```python
from build123d import *

# Parameters (mm, degrees)
SKETCH1_W           = 20
SKETCH1_H           = 80
BOSS_EXTRUDE1_DEPTH = 20
SKETCH2_R           = 5
CUT_EXTRUDE1_DEPTH  = 49.989794856
SKETCH5_R           = 3.175
CUT_EXTRUDE4_DEPTH  = 49.989794856
CUT_EXTRUDE3_DEPTH  = 5


with BuildPart() as part:
    # Sketch1 → Boss-Extrude1 (new body)
    with BuildSketch(Plane(origin=(0, 0, 0), x_dir=(1, 0, 0), z_dir=(0, 1, 0))):
        Rectangle(SKETCH1_W, SKETCH1_H)
    extrude(amount=BOSS_EXTRUDE1_DEPTH)

    # Sketch2 → Cut-Extrude1 (cut, through all)
    with BuildSketch(Plane(origin=(10, 0, 0), x_dir=(0, 0, -1), z_dir=(1, 0, 0))):
        with Locations((-20, 10)):
            Circle(SKETCH2_R)
        with Locations(Location((20, 10, 0), (0, 0, 180))):
            Circle(SKETCH2_R)
    extrude(amount=-CUT_EXTRUDE1_DEPTH, mode=Mode.SUBTRACT)

    # Sketch5 → Cut-Extrude4 (cut, through all)
    with BuildSketch(Plane(origin=(10, 0, 0), x_dir=(0, 0, -1), z_dir=(1, 0, 0))):
        with Locations((0, 10)):
            Circle(SKETCH5_R)
    extrude(amount=-CUT_EXTRUDE4_DEPTH, mode=Mode.SUBTRACT)

    # Sketch3 → Cut-Extrude3 (cut)
    with BuildSketch(Plane(origin=(10, 0, 0), x_dir=(0, 0, -1), z_dir=(1, 0, 0))):
        Polygon((0, 16), (-5.196152423, 13), (-5.196152423, 7), (0, 4), (5.196152423, 7), (5.196152423, 13), align=None)
    cut_extrude3 = extrude(amount=-CUT_EXTRUDE3_DEPTH, mode=Mode.SUBTRACT)

    # Mirror1: Cut-Extrude3 across plane
    add(cut_extrude3.mirror(Plane(origin=(0, 0, 0), x_dir=(0, 0, 1), z_dir=(1, 0, 0))), mode=Mode.SUBTRACT)


solid = part.part
```
The model under review builds one solid part; all positions refer to its coordinate system, in mm. A direction names the side the tool comes from. Give positions to 0.01 mm unless a question says otherwise; leave off trailing zeros. Write each loop counter-clockwise with the first axis right and the second up, starting at its lowest first coordinate (ties: lowest second). Pieces come first, ordered by that corner, then holes. Notation, with made-up numbers: (-27.5, -17.75) -> (5.5, -17.75) arc R18 ccw to (5.5, 1.25) -> close; hole circle Ø5 at (-39.75, 50.25). An arc over 180 degrees is marked (long way). Put each result on its own line as item: value.
(1) For pin 1 Ø3 at (y, z) = (9.5, -2) entering from +X; pin 2 Ø8.5 at (y, z) = (10.5, -0.5) entering from -X, all flat-tipped, find the tip position at first contact; note any pin that passes through.
Results are:
pin 1: x = 5
pin 2: x = -5
(2) Tool access review of faces 4 (the flat face through (-8, 10, -5.196)), 5 (the flat face through (-10, 3, 1)), 6 (the flat face through (7.5, 14.5, -2.6)): name each direction out of +Z, -Z, +X, -X, +Y, -Y from which nothing blocks a thin tool from reaching the whole face with its end or side.
Results are:
face 4: -X
face 5: +Z, -Z, -X, +Y, -Y
face 6: +X
(3) We need section A-A, the plane y = 10. Give the boundary of the cut face in (x, z) (3 decimals), and give its area (3 significant figures).
Results are:
outline: (-10, -40) -> (10, -40) -> (10, -25) -> (-10, -25) -> close; (-10, -15) -> (10, -15) -> (10, -5.196) -> (5, -5.196) -> (5, -3.175) -> (-5, -3.175) -> (-5, -5.196) -> (-10, -5.196) -> close; (-10, 5.196) -> (-5, 5.196) -> (-5, 3.175) -> (5, 3.175) -> (5, 5.196) -> (10, 5.196) -> (10, 15) -> (-10, 15) -> close; (-10, 25) -> (10, 25) -> (10, 40) -> (-10, 40) -> close
area: 1,030 mm²
(4) The part is to be moulded in two halves that separate along Z. For faces 1 (the flat face through (5, 7, 2)), 2 (the flat face through (0, 10, -40)), 3 (the flat face through (0, 0, -1)), say which applies: pulls with the +Z half, pulls with the -Z half, needs draft (parallel to the pull), parting line crosses it, or undercut.
Results are:
face 1: undercut
face 2: pulls with the -Z half
face 3: needs draft
(5) We need section B-B, the plane x = 8.5. Give the boundary of the cut face in (y, z).
Results are:
outline: (0, -40) -> (20, -40) -> (20, 40) -> (0, 40) -> close; hole (4, 0) -> (7, -5.2) -> (13, -5.2) -> (16, 0) -> (13, 5.2) -> (7, 5.2) -> close; hole circle Ø10 at (10, -20); hole circle Ø10 at (10, 20)
(6) To check wall thickness, follow probe 1 along Y at (x, z) = (-7.75, 20); probe 2 along Z at (x, y) = (-3, 6.5); probe 3 along Y at (x, z) = (3.25, 0) (3 decimals). State the ranges of each line that lie inside material, in increasing order. Write a range as from..to.
Results are:
probe 1: 0..5, 15..20
probe 2: -40..-23.57, -16.43..16.43, 23.57..40
probe 3: 0..6.825, 13.175..20
(7) We need section C-C, the plane z = 20. Give the boundary of the cut face in (x, y), and give its area (3 significant figures).
Results are:
outline: (-10, 0) -> (10, 0) -> (10, 5) -> (-10, 5) -> close; (-10, 15) -> (10, 15) -> (10, 20) -> (-10, 20) -> close
area: 200 mm²
(8) We need section D-D, the plane z = -4. Give the boundary of the cut face in (x, y), and give its area (3 significant figures).
Results are:
outline: (-10, 0) -> (10, 0) -> (10, 6.31) -> (5, 6.31) -> (5, 13.69) -> (10, 13.69) -> (10, 20) -> (-10, 20) -> (-10, 13.69) -> (-5, 13.69) -> (-5, 6.31) -> (-10, 6.31) -> close
area: 326 mm²
